CAD build for the part. Positions are in the model's coordinates, mm. Give positions to 0.01 mm unless a question says otherwise; leave off trailing zeros. Loops run counter-clockwise (first coordinate to the right, second up) from the corner with the lowest first, then second, coordinate; pieces in that order, holes last. Notation, with made-up numbers: (31, 17.5) -> (69, 17.5) arc R15 ccw to (69, 26.5) -> close; hole circle Ø3 at (55, 20). An arc over 180 degrees is marked (long way). Use one line per item in the form item = value.
```python
from build123d import *

# Parameters (mm, degrees)
F0_R     = 11
F1_DEPTH = 12


with BuildPart() as f1:
    # F0 (on Top) → F1 (new body)
    with BuildSketch(Plane.XY):
        with BuildLine():
            ThreePointArc((-62.5, -29.5), (-61.035534, -33.035534), (-57.5, -34.5))
            Line((-57.5, -34.5), (57.5, -34.5))
            ThreePointArc((57.5, -34.5), (61.035534, -33.035534), (62.5, -29.5))
            Line((62.5, -29.5), (62.5, 34.5))
            Line((62.5, 34.5), (-62.5, 34.5))
            Line((-62.5, 34.5), (-62.5, -29.5))
        make_face()
        with Locations((-32.5, 0)):
            Circle(F0_R, mode=Mode.SUBTRACT)
        with Locations((32.5, 0)):
            Circle(F0_R, mode=Mode.SUBTRACT)
    extrude(amount=F1_DEPTH)


solid = f1.part
```
1. Drill centre lines: line 1 (Y direction, x = 32.5, z = 8.5); line 2 (X direction, y = 3, z = 10); line 3 (X direction, y = -8.5, z = 7.25). Where is each one in solid material? Low to high.
Result sheet:
line_1 = -34.5 to -11, 11 to 34.5
line_2 = -62.5 to -43.08, -21.92 to 21.92, 43.08 to 62.5
line_3 = -62.5 to -39.48, -25.52 to 25.52, 39.48 to 62.5
2. Cut at C-C, the plane z = 7.5. Write the cut outline in (x, y).
Result sheet:
outline = (-62.5, -29.5) arc R5 ccw to (-57.5, -34.5) -> (57.5, -34.5) arc R5 ccw to (62.5, -29.5) -> (62.5, 34.5) -> (-62.5, 34.5) -> close; hole circle Ø22 at (-32.5, 0); hole circle Ø22 at (32.5, 0)
3. Cut at D-D, the plane x = 35. Write the cut outline in (y, z).
Result sheet:
outline = (-34.5, 0) -> (-10.71, 0) -> (-10.71, 12) -> (-34.5, 12) -> close; (10.71, 0) -> (34.5, 0) -> (34.5, 12) -> (10.71, 12) -> close
4. Cut at B-B, the plane y = 0. Write the cut outline in (x, z), then the cut area to 3 significant figures.
Result sheet:
outline = (-62.5, 0) -> (-43.5, 0) -> (-43.5, 12) -> (-62.5, 12) -> close; (-21.5, 0) -> (21.5, 0) -> (21.5, 12) -> (-21.5, 12) -> close; (43.5, 0) -> (62.5, 0) -> (62.5, 12) -> (43.5, 12) -> close
area = 972 mm^2
5. Cut at A-A, the plane x = -32.5. Write the cut outline in (y, z).
Result sheet:
outline = (-34.5, 0) -> (-11, 0) -> (-11, 12) -> (-34.5, 12) -> close; (11, 0) -> (34.5, 0) -> (34.5, 12) -> (11, 12) -> close
6. Mould opens along Y. For faces 1 (the flat face through (-1, 0, 12)), 2 (the cylindrical face through (-61.07, -33, 5.92)), 3 (the cylindrical face through (-22.339, -4.213, 5.916)) say: pulls with the +Y half, pulls with the -Y half, needs draft (parallel to the pull), parting line crosses it, or undercut.
Result sheet:
face_1 = needs draft
face_2 = pulls with the -Y half
face_3 = undercut
